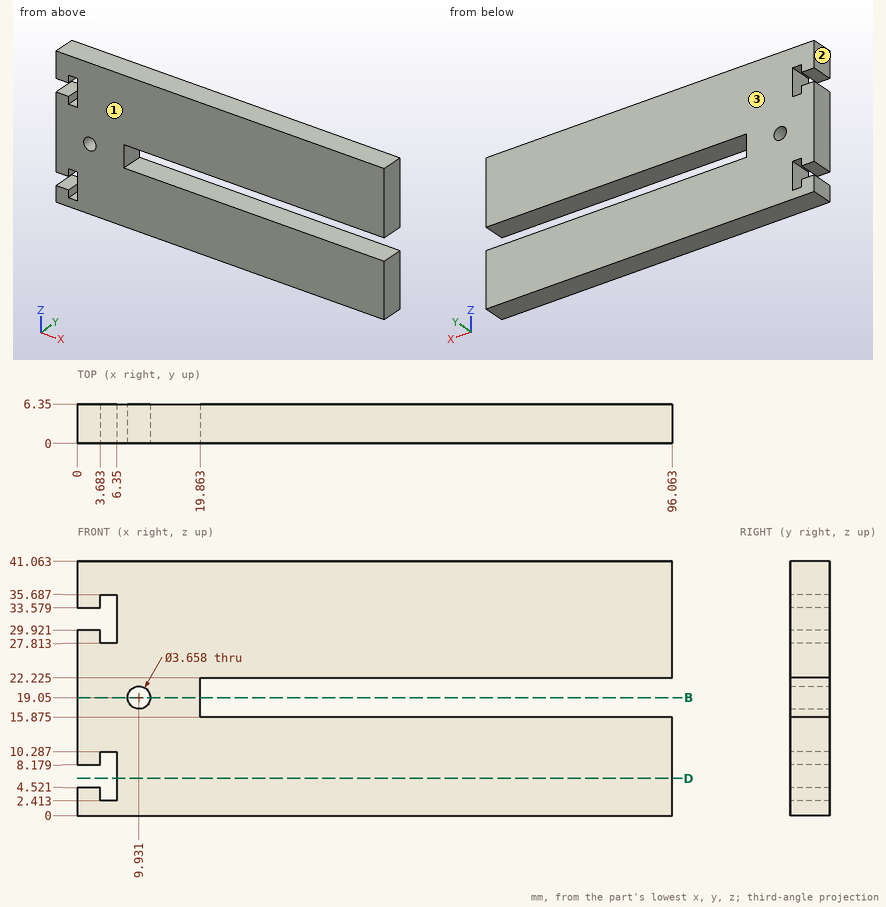
Study the drawing (mm; zero at the part's minimum x, y, z) and answer. Round coordinates to 2 decimals unless told otherwise and drop trailing zeros. Write each loop counter-clockwise with the first axis right and the second up, starting at its lowest first coordinate (ties: lowest second). Pieces come first, ordered by that corner, then holes.
Q1. A flat-ended cylindrical pin translates along its axis: P1, Ø1.9, axis at y = 3, z = 20, coming from the +X side. Find the tip coordinate at first contact, or state that the pin passes through.
Values:
P1: stops at x = 19.86
Q2. Straight lines are drawn through the part: line 1 (Z direction, x = 73, y = 4) (1 decimal); line 2 (X direction, y = 0.5, z = 6); line 3 (X direction, y = 5.5, z = 34). For each, find the intervals that lie inside material, in ascending order.
Values:
line 1: z = 0 to 15.9, 22.2 to 41.1
line 2: x = 6.35 to 96.06
line 3: x = 0 to 3.68, 6.35 to 96.06
Q3. The mould has two halves that part along Y. Classify the marked faces 1, 2 and 3: released by +Y, released by -Y, zero draft, split by the parting line, or undercut.
Values:
face 1: released by -Y
face 2: zero draft
face 3: released by +Y
Q4. Find section D-D on z = 6. Determine the outline of the cut face in (x, y).
Values:
outline: (6.35, 0) - (96.06, 0) - (96.06, 6.35) - (6.35, 6.35) - close
Q5. Find section B-B on z = 19.05. Determine the outline of the cut face in (x, y), and give its area (3 significant figures).
Values:
outline: (0, 0) - (8.1, 0) - (8.1, 6.35) - (0, 6.35) - close; (11.76, 0) - (19.86, 0) - (19.86, 6.35) - (11.76, 6.35) - close
area: 103 mm2
